from build123d import *

# Parameters (mm, degrees)
F1_DEPTH = 0.75
F2_DEPTH = 1.2
F3_DEPTH = 0.5
F4_R     = 1.5
F5_DEPTH = 1


with BuildPart() as f1:
    # F0 (on Top) → F1 (new body)
    with BuildSketch(Plane.XY):
        Polygon((17, 0), (0, 30), (-17, 0), align=None)
        Polygon((-9.8602514396, 10.5712104419), (0, 27.9716541589), (9.8602514396, 10.5712104419), (6.91278449, 9.2867956266), (13.8255689799, 3.5735912532), (15.2839373567, 1), (12.2839373567, 1), (-12.2839373567, 1), (-15.2839373567, 1), (-13.7839373567, 3.5980762114), (-6.8919686783, 9.2990381057), align=None, mode=Mode.SUBTRACT)
    extrude(amount=F1_DEPTH)



with BuildPart() as f1b:
    # F0 (on Top) → F1, piece 2 (new body)
    with BuildSketch(Plane.XY):
        with BuildLine():
            Line((4.2646633267, 16.3890860177), (0, 23.9149624766))
            Line((0, 23.9149624766), (-4.2646633267, 16.3890860177))
            ThreePointArc((-4.2646633267, 16.3890860177), (0, 17), (4.2646633267, 16.3890860177))
        make_face()
    extrude(amount=F1_DEPTH)


with BuildPart() as f1c:
    # F0 (on Top) → F1, piece 3 (new body)
    with BuildSketch(Plane.XY):
        with BuildLine():
            ThreePointArc((-2, 14.8474978515), (-4.53528859, 14.1958216086), (-6.8919686783, 13.0563352674))
            Line((-6.8919686783, 13.0563352674), (-5.0466307357, 10.8254816785))
            Line((-5.0466307357, 10.8254816785), (-1.5410891317, 13.7252277505))
            ThreePointArc((-1.5410891317, 13.7252277505), (-1.3920172008, 14.4411475731), (-2, 14.8474978515))
        make_face()
    extrude(amount=F1_DEPTH)


with BuildPart() as f1d:
    # F0 (on Top) → F1, piece 4 (new body)
    with BuildSketch(Plane.XY):
        with BuildLine():
            Line((5.049368775, 10.8268515661), (6.8919686783, 13.0563352674))
            ThreePointArc((6.8919686783, 13.0563352674), (4.53528859, 14.1958216086), (2, 14.8474978515))
            ThreePointArc((2, 14.8474978515), (1.3921371588, 14.4414464477), (1.5416340213, 13.7258867616))
            Line((1.5416340213, 13.7258867616), (5.049368775, 10.8268515661))
        make_face()
    extrude(amount=F1_DEPTH)


with BuildPart() as f1e:
    # F0 (on Top) → F1, piece 5 (new body)
    with BuildSketch(Plane.XY):
        Polygon((0, 11), (-2.997756418, 8.5596127439), (0, 7.2146742605), (2.927840303, 8.6165294417), align=None)
    extrude(amount=F1_DEPTH)


with BuildPart() as f1f:
    # F0 (on Top) → F1, piece 6 (new body)
    with BuildSketch(Plane.XY):
        Polygon((-4.5487910115, 7.2969601038), (-9.097582023, 3.5939202075), (-1, 3.5867390231), (-1, 5.5867390231), align=None)
    extrude(amount=F1_DEPTH)


with BuildPart() as f1g:
    # F0 (on Top) → F1, piece 7 (new body)
    with BuildSketch(Plane.XY):
        Polygon((1, 5.5849653616), (1, 3.5849653616), (9.117425038, 3.5777665798), (4.558712519, 7.2888832899), align=None)
    extrude(amount=F1_DEPTH)


with BuildPart() as f1_1:
    add(f1.part)

    add(f1b.part)  # F2 merges F1b

    add(f1c.part)  # F2 merges F1c

    add(f1d.part)  # F2 merges F1d

    add(f1e.part)  # F2 merges F1e

    add(f1f.part)  # F2 merges F1f

    add(f1g.part)  # F2 merges F1g
    # F0 (on Top) → F2 (join)
    with BuildSketch(Plane.XY):
        with BuildLine():
            Line((9.8602514396, 10.5712104419), (0, 27.9716541589))
            Line((0, 27.9716541589), (-9.8602514396, 10.5712104419))
            ThreePointArc((-9.8602514396, 10.5712104419), (-8.467773088, 11.9232570085), (-6.8919686783, 13.0563352674))
            ThreePointArc((-6.8919686783, 13.0563352674), (-4.53528859, 14.1958216086), (-2, 14.8474978515))
            ThreePointArc((-2, 14.8474978515), (-1.3920172008, 14.4411475731), (-1.5410891317, 13.7252277505))
            Line((-1.5410891317, 13.7252277505), (-5.0466307357, 10.8254816785))
            Line((-5.0466307357, 10.8254816785), (-6.8919686783, 9.2990381057))
            Line((-6.8919686783, 9.2990381057), (-13.7839373567, 3.5980762114))
            Line((-13.7839373567, 3.5980762114), (-12.2839373567, 1))
            Line((-12.2839373567, 1), (12.2839373567, 1))
            Line((12.2839373567, 1), (13.8255689799, 3.5735912532))
            Line((13.8255689799, 3.5735912532), (6.91278449, 9.2867956266))
            Line((6.91278449, 9.2867956266), (5.049368775, 10.8268515661))
            Line((5.049368775, 10.8268515661), (1.5416340213, 13.7258867616))
            ThreePointArc((1.5416340213, 13.7258867616), (1.3921371588, 14.4414464477), (2, 14.8474978515))
            ThreePointArc((2, 14.8474978515), (4.53528859, 14.1958216086), (6.8919686783, 13.0563352674))
            ThreePointArc((6.8919686783, 13.0563352674), (8.467773088, 11.9232570085), (9.8602514396, 10.5712104419))
        make_face()
        Polygon((-1, 3.5867390231), (-9.097582023, 3.5939202075), (-4.5487910115, 7.2969601038), (-2.997756418, 8.5596127439), (0, 11), (2.927840303, 8.6165294417), (4.558712519, 7.2888832899), (9.117425038, 3.5777665798), (1, 3.5849653616), align=None, mode=Mode.SUBTRACT)
        with BuildLine():
            Line((-4.2646633267, 16.3890860177), (0, 23.9149624766))
            Line((0, 23.9149624766), (4.2646633267, 16.3890860177))
            ThreePointArc((4.2646633267, 16.3890860177), (0, 17), (-4.2646633267, 16.3890860177))
        make_face(mode=Mode.SUBTRACT)
    extrude(amount=F2_DEPTH)

    # F0 (on Top) → F3 (join)
    with BuildSketch(Plane.XY):
        with BuildLine():
            ThreePointArc((-6.8919686783, 13.0563352674), (-8.467773088, 11.9232570085), (-9.8602514396, 10.5712104419))
            Line((-9.8602514396, 10.5712104419), (-6.8919686783, 9.2990381057))
            Line((-6.8919686783, 9.2990381057), (-5.0466307357, 10.8254816785))
            Line((-5.0466307357, 10.8254816785), (-6.8919686783, 13.0563352674))
        make_face()
        Polygon((-1, 5.5867390231), (-1, 3.5867390231), (1, 3.5849653616), (1, 5.5849653616), (4.558712519, 7.2888832899), (2.927840303, 8.6165294417), (0, 7.2146742605), (-2.997756418, 8.5596127439), (-4.5487910115, 7.2969601038), align=None)
        with BuildLine():
            Line((6.91278449, 9.2867956266), (9.8602514396, 10.5712104419))
            ThreePointArc((9.8602514396, 10.5712104419), (8.467773088, 11.9232570085), (6.8919686783, 13.0563352674))
            Line((6.8919686783, 13.0563352674), (5.049368775, 10.8268515661))
            Line((5.049368775, 10.8268515661), (6.91278449, 9.2867956266))
        make_face()
    extrude(amount=F3_DEPTH)

    # F4
    f4_edges = [f1_1.edges().sort_by_distance(p)[0] for p in [
        (0, 30, 0.375),
        (-17, 0, 0.375),
        (17, 0, 0.375),
    ]]
    fillet(f4_edges, radius=F4_R)

    # F0 (on Top) → F5 (join)
    with BuildSketch(Plane.XY):
        Polygon((-12.2839373567, 1), (-13.7839373567, 3.5980762114), (-15.2839373567, 1), align=None)
        Polygon((15.2839373567, 1), (13.8255689799, 3.5735912532), (12.2839373567, 1), align=None)
    extrude(amount=F5_DEPTH)


solid = f1_1.part
Could you check a few things on this model? Use its own coordinates, in mm. A direction names the side the tool comes from. Give positions to 0.01 mm unless a question says otherwise; leave off trailing zeros. Loops run counter-clockwise (first coordinate to the right, second up) from the corner with the lowest first, then second, coordinate; pieces in that order, holes last. Notation, with made-up numbers: (-10.5, 82) -> (16.5, 82) arc R26 ccw to (16.5, 108) -> close; hole circle Ø10 at (17, 64). An arc over 180 degrees is marked (long way). Return JSON: item names as keys, results as strings.
Item 1: If we section it at C-C on x = -8: List the corners of the cut face in (y, z) for me, plus the area to 3 significant figures.
Geometry results:
{"outline": "(0, 0) -> (15.88, 0) -> (15.88, 0.75) -> (13.85, 0.75) -> (13.85, 1.2) -> (12.3, 1.2) -> (12.3, 0.5) -> (9.77, 0.5) -> (9.77, 0.75) -> (8.38, 0.75) -> (8.38, 1.2) -> (4.49, 1.2) -> (4.49, 0.75) -> (3.59, 0.75) -> (3.59, 1.2) -> (1, 1.2) -> (1, 0.75) -> (0, 0.75) -> close", "area": "14.9 mm²"}
Item 2: Which directions (+Z, -Z, +X, -X, +Y, -Y) give clear straight access to the entire face, cutting with the end or side of a thin tool? Please do faces 1 (the flat face through (-4.861, 19.393, 0.972)), 2 (the flat face through (2.102, 20.205, 0.972)), 3 (the flat face through (-8.417, 15.146, 0.37)).
Geometry results:
{"face 1": "+Z, -X, +Y", "face 2": "+Z", "face 3": "+Z, -Z, -X, +Y"}
Item 3: I need wall thicknesses on L1, parallel to Y at x = -4, z = 1.1; L2, parallel to Y at x = -5, z = 1; L3, parallel to Y at x = 2.5, z = 1.1. Which ranges of each line are inside material? Lowest first, please. Write a range as from..to.
Geometry results:
{"L1": "y = 1..3.59, 7.74..11.69, 14.38..16.46, 16.86..20.91", "L2": "y = 1..3.59, 6.93..10.86, 14.02..19.15", "L3": "y = 1..3.58, 8.96..12.93, 14.76..16.79, 19.5..23.56"}
Item 4: We'd pull the mould along Y, two halves only. Please class faces 4 (the cylindrical face through (-15.73, 0.76, 0.38)), 5 (the flat face through (-14, 2, 1)), 6 (the flat face through (-2.16, 20.1, 0.97)): +Y half, -Y half, draft (parallel to the pull), parting line (faces both ways), or undercut.
Geometry results:
{"face 4": "parting line", "face 5": "draft", "face 6": "undercut"}
Item 5: If we section it at B-B on y = 25: List the corners of the cut face in (x, z) for me.
Geometry results:
{"outline": "(-2.83, 0) -> (2.83, 0) -> (2.83, 0.75) -> (1.68, 0.75) -> (1.68, 1.2) -> (-1.68, 1.2) -> (-1.68, 0.75) -> (-2.83, 0.75) -> close"}
Item 6: I'm going to push flat-ended pins straight in: pin 1 (1.1 mm diameter, centred on x = -7, y = 10.5, fed in from +Z); pin 2 (1.5 mm diameter, centred on x = 2, y = 5.5, fed in from +Z). Where does each tip first touch, or does it pass through?
Geometry results:
{"pin 1": "stops at z = 0.5", "pin 2": "stops at z = 0.75"}
Item 7: If we section it at A-A on z = 0.2: List the corners of the cut face in (x, y) for me.
Geometry results:
{"outline": "(-15.73, 2.24) arc R1.5 ccw to (-14.43, 0) -> (14.43, 0) arc R1.5 ccw to (15.73, 2.24) -> (1.31, 27.7) arc R1.5 ccw to (-1.31, 27.7) -> close"}
Item 8: If we section it at D-D on y = 4: List the corners of the cut face in (x, z) for me.
Geometry results:
{"outline": "(-14.73, 0) -> (14.73, 0) -> (14.73, 0.75) -> (13.31, 0.75) -> (13.31, 1.2) -> (8.6, 1.2) -> (8.6, 0.75) -> (1, 0.75) -> (1, 0.5) -> (-1, 0.5) -> (-1, 0.75) -> (-8.6, 0.75) -> (-8.6, 1.2) -> (-13.3, 1.2) -> (-13.3, 0.75) -> (-14.73, 0.75) -> close"}
